Check sheet for the drawn part. Datum: minimum x, y, z corner. Units: mm. A direction names the side the tool comes from. Coordinates: 2 decimals unless noted, no trailing zeros. Write each loop counter-clockwise with the first axis right and the second up, starting at its lowest first coordinate (ties: lowest second). Pieces come first, ordered by that corner, then holes. Notation, with made-up numbers: (-13.75, -4) -> (9.25, -4) arc R14 cw to (9.25, 12) -> close; hole circle Ø2 at (49, -5.75). An arc over 180 degrees is marked (long way). Answer in a Markdown table with one row per item.
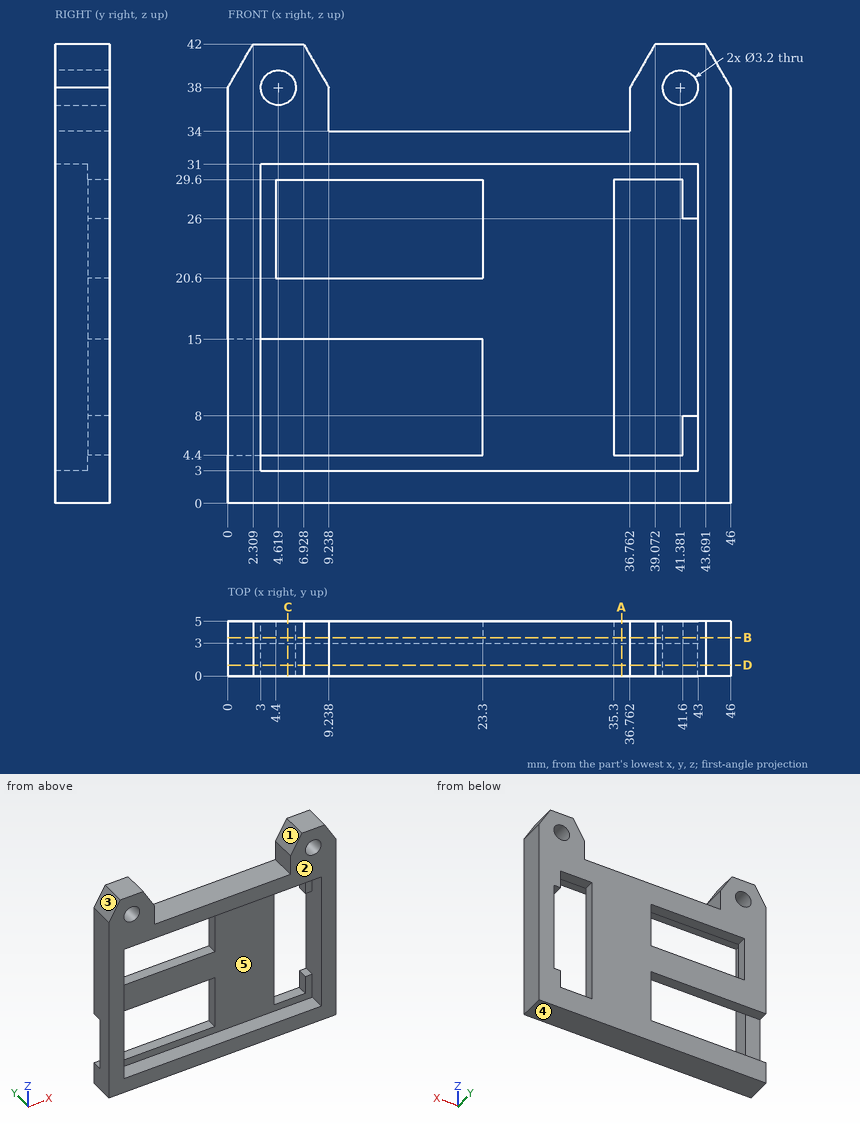
1. Go/stop test with flat-tipped pins: pin 1 (1.5 mm diameter, centred on x = 17, y = 1.5, fed in from +Z); pin 2 (1.5 mm diameter, centred on x = 2, z = 7.5, fed in from +Y); pin 3 (2 mm diameter, centred on x = 41, z = 10.5, fed in from +Y); pin 4 (8.5 mm diameter, centred on x = 15, z = 15.5, fed in from -Y). Record where each tip stops, or that it passes through.
Findings below:
| item | result |
|---|---|
| pin 1 | stops at z = 34 |
| pin 2 | stops at y = 3 |
| pin 3 | passes through |
| pin 4 | stops at y = 3 |
2. Release check for a two-part mould opening along X. For the marked faces 3, 4 and 5 record: released by +X, released by -X, zero draft, split by the parting line, or undercut.
Findings below:
| item | result |
|---|---|
| face 3 | released by -X |
| face 4 | zero draft |
| face 5 | undercut |
3. Sectioned sample at A-A, the plane x = 36. Record the cut outline in (y, z).
Findings below:
| item | result |
|---|---|
| outline | (0, 0) -> (5, 0) -> (5, 4.4) -> (3, 4.4) -> (3, 3) -> (0, 3) -> close; (0, 31) -> (3, 31) -> (3, 29.6) -> (5, 29.6) -> (5, 34) -> (0, 34) -> close |
4. Sectioned sample at D-D, the plane y = 1. Record the cut outline in (x, z).
Findings below:
| item | result |
|---|---|
| outline | (0, 0) -> (46, 0) -> (46, 38) -> (43.69, 42) -> (39.07, 42) -> (36.76, 38) -> (36.76, 34) -> (9.24, 34) -> (9.24, 38) -> (6.93, 42) -> (2.31, 42) -> (0, 38) -> close; hole (3, 3) -> (43, 3) -> (43, 31) -> (3, 31) -> close; hole circle Ø3.2 at (4.62, 38); hole circle Ø3.2 at (41.38, 38) |
5. Access from +Z, -Z, +X, -X, +Y, -Y to the whole of each face (thin tool, end or side, straight path). Record for the marked faces 1 and 2.
Findings below:
| item | result |
|---|---|
| face 1 | +Z, +Y, -Y |
| face 2 | +Z, -Z, +X, -X, -Y |
6. Sectioned sample at B-B, the plane y = 3.5. Count the separate pieces of the cut face and the enclosed holes in it, and give its area (3 significant figures).
Findings below:
| item | result |
|---|---|
| separate pieces | 1 |
| enclosed holes | 4 |
| area | 1,080 mm² |
7. Material ranges on probe 1 along X at (y, z) = (2.15, 38); probe 2 along X at (y, z) = (3.05, 26.5); probe 3 along X at (y, z) = (3.25, 24), recorded low to high. Write a range as from..to.
Findings below:
| item | result |
|---|---|
| probe 1 | x = 0..3.02, 6.22..9.24, 36.76..39.78, 42.98..46 |
| probe 2 | x = 0..4.4, 23.3..35.3, 41.6..46 |
| probe 3 | x = 0..4.4, 23.3..35.3, 43..46 |
8. Sectioned sample at C-C, the plane x = 5.5. Record the cut outline in (y, z) (1 decimal).
Findings below:
| item | result |
|---|---|
| outline | (0, 0) -> (5, 0) -> (5, 4.4) -> (3, 4.4) -> (3, 3) -> (0, 3) -> close; (0, 31) -> (3, 31) -> (3, 29.6) -> (5, 29.6) -> (5, 36.7) -> (0, 36.7) -> close; (0, 39.3) -> (5, 39.3) -> (5, 42) -> (0, 42) -> close; (3, 15) -> (5, 15) -> (5, 20.6) -> (3, 20.6) -> close |
